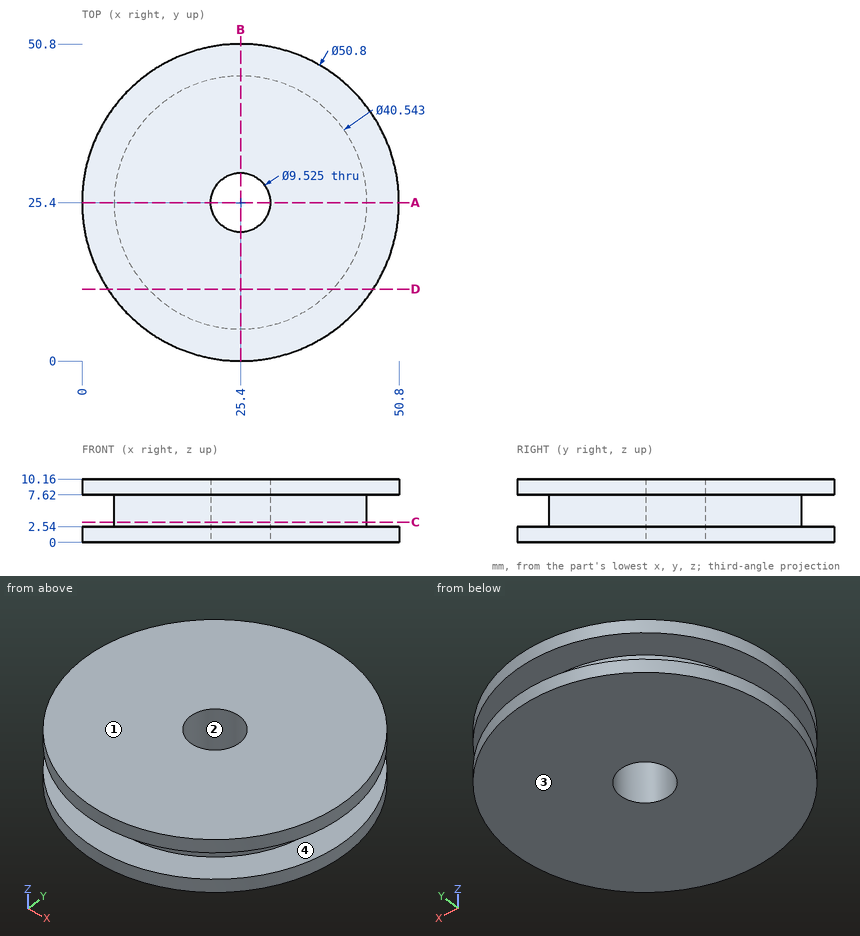
For this review, use the dimensioned drawing (mm, ordinates from the lowest corner) and the shaded views. A direction names the side the tool comes from. Round coordinates to 2 decimals unless told otherwise and drop trailing zeros. Order: outer loops, then holes, each group sorted by start corner. A loop starts at its lowest first (then second) coordinate and runs counter-clockwise, first axis right, second up. Notation, with made-up numbers: (25.5, 31.25) -> (77.5, 31.25) arc R30 ccw to (77.5, 54.25) -> close; hole circle Ø3 at (6.5, 34). An arc over 180 degrees is marked (long way). Use CSV: the item, a comma, the result in double quotes. Start each with the question number.
(1) Wall thickness on probe 1 along Y at (x, z) = (25.4, 3.75); probe 2 along Z at (x, y) = (6.5, 36.5); probe 3 along X at (y, z) = (31, 5.5): over which ranges is each line inside the solid? List them lowest first. Write a range as from..to.
(2) Consider section A-A on y = 25.4. Write out the cut boundary in (x, z).
(3) Mouldability with a two-part tool opening along X and no side actions: class the marked faces 1 and 2 as pulls with the +X half, pulls with the -X half, needs draft (parallel to the pull), parting line crosses it, or undercut.
(4) Consider section C-C on z = 3.25. Write out the cut boundary in (x, y) (1 decimal), and give its area (3 significant figures).
(5) Consider section D-D on y = 11.5. Write out the cut boundary in (x, z).
(6) Insertion check: pin 1 (1 mm diameter, centred on x = 18, z = 2, fed in from +Y) (1 decimal); pin 2 (1 mm diameter, centred on x = 31.5, z = 1, fed in from +Y) (3 decimals); pin 3 (6 mm diameter, centred on x = 9, z = 3, fed in from +Y). Each pin has a flat end and moves straight along its axis. Give the tip position at first contact, or say it passes through.
(7) Tool access review of the marked faces 3 and 4: name each direction out of +Z, -Z, +X, -X, +Y, -Y from which nothing blocks a thin tool from reaching the whole face with its end or side.
Responses:
1,probe 1,"5.13..20.64, 30.16..45.67"
1,probe 2,"0..2.54, 7.62..10.16"
1,probe 3,"5.92..44.88"
2,outline,"(0, 0) -> (20.64, 0) -> (20.64, 10.16) -> (0, 10.16) -> (0, 7.62) -> (5.13, 7.62) -> (5.13, 2.54) -> (0, 2.54) -> close; (30.16, 0) -> (50.8, 0) -> (50.8, 2.54) -> (45.67, 2.54) -> (45.67, 7.62) -> (50.8, 7.62) -> (50.8, 10.16) -> (30.16, 10.16) -> close"
3,face 1,"needs draft"
3,face 2,"undercut"
4,outline,"circle Ø40.5 at (25.4, 25.4); hole circle Ø9.5 at (25.4, 25.4)"
4,area,"1,220 mm²"
5,outline,"(4.14, 0) -> (46.66, 0) -> (46.66, 2.54) -> (40.16, 2.54) -> (40.16, 7.62) -> (46.66, 7.62) -> (46.66, 10.16) -> (4.14, 10.16) -> (4.14, 7.62) -> (10.64, 7.62) -> (10.64, 2.54) -> (4.14, 2.54) -> close"
6,pin 1,"y = 49.8"
6,pin 2,"y = 50.175"
6,pin 3,"y = 46.96"
7,face 3,"-Z, +X, -X, +Y, -Y"
7,face 4,"none"
